Model file for the job. Use its own axes, mm. A direction names the side the tool comes from. Round coordinates to 2 decimals unless told otherwise and drop trailing zeros. Order: outer loops, then holes, each group sorted by start corner. A loop starts at its lowest first (then second) coordinate and runs counter-clockwise, first axis right, second up. Notation, with made-up numbers: (-8, 64) - (19, 64) arc R14 ccw to (19, 78) - close; hole circle Ø3 at (22, 87). An arc over 180 degrees is marked (long way). Answer as CSV lines item,"result". Start each with the question number.
1. Band-saw the part on C-C on y = -11.75. List the corners of the cut face in (x, z), then the cut area to 3 significant figures.
2. Pull direction X, two halves, no side cores. Call faces 6 (the face through (41.668, -11.944, 0.084)), 7 (the face through (-6, -4, 0)), 8 (the face through (77, -8, 0)): released by +X, released by -X, zero draft, split by the parting line, or undercut.
3. Band-saw the part on A-A on x = 85. List the corners of the cut face in (y, z).
4. Pin check, flat tips, straight feed: pin 1 Ø8 at (x, y) = (49.5, -6) entering from -Z; pin 2 Ø7.5 at (x, z) = (-2, -0.5) entering from -Y; pin 3 Ø2 at (x, z) = (60, -4) entering from +Y; pin 4 Ø12 at (x, z) = (30.5, 1) entering from +Y. Stop position of each tip, or through.
5. Band-saw the part on B-B on z = 5. List the corners of the cut face in (x, y), then the cut area to 3 significant figures.
6. Wall check: line 1 along Z through (x, y) = (85, -13.5); line 2 along Z through (x, y) = (0, -2); line 3 along Z through (x, y) = (18, -7.5). Give the ranges that are in metal, low to high. Write a range as [from, to].
7. 3-axis set-ups, long thin cutter, end or side, ignore diameter. For faces 1 (the face through (76, -16, 0)), 2 (the face through (44, -8, -6)), 3 (the face through (76.39, -12.06, 6.47)), 4 (the face through (7, -8, 0)), 5 (the face through (45, -8, 6)): which of +Z, -Z, +X, -X, +Y, -Y reach the whole face in a straight line?
8. Band-saw the part on D-D on x = 0. List the corners of the cut face in (y, z).
```python
from build123d import *

# Parameters (mm, degrees)
F0_R     = 6
F1_DEPTH = 25
F3_DEPTH = 12.5
F4_R     = 8


with BuildPart() as f1:
    # F0 (on Front) → F1 (new body)
    with BuildSketch(Plane.XZ):
        with BuildLine():
            ThreePointArc((10.965856, -6), (12.110392, -3.096514), (12.5, 0))
            ThreePointArc((12.5, 0), (12.110392, 3.096514), (10.965856, 6))
            ThreePointArc((10.965856, 6), (-12.5, 0), (10.965856, -6))
        make_face()
        Circle(F0_R, mode=Mode.SUBTRACT)
        with BuildLine():
            ThreePointArc((10.965856, 6), (12.110392, 3.096514), (12.5, 0))
            ThreePointArc((12.5, 0), (12.110392, -3.096514), (10.965856, -6))
            Line((10.965856, -6), (77, -6))
            ThreePointArc((77, -6), (75, 0), (77, 6))
            Line((77, 6), (10.965856, 6))
        make_face()
        with BuildLine():
            ThreePointArc((95, 0), (88.162278, 9.486833), (77, 6))
            ThreePointArc((77, 6), (75, 0), (77, -6))
            ThreePointArc((77, -6), (88.162278, -9.486833), (95, 0))
        make_face()
        with Locations((85, 0)):
            Circle(F0_R, mode=Mode.SUBTRACT)
    extrude(amount=F1_DEPTH)

    # F2 (on Top) → F3 (intersect, symmetric)
    with BuildSketch(Plane.XY):
        Polygon((20, 0), (-12.5, 0), (-12.5, -8), (19.300091, -8), (64.670345, -16), (95, -16), (95, -8), (65.370255, -8), align=None)
    extrude(amount=F3_DEPTH, both=True, mode=Mode.INTERSECT)

    # F4
    f4_edges = [f1.edges().sort_by_distance(p)[0] for p in [
        (10.965856, -4, -6),
        (10.965856, -4, 6),
        (77, -12, 6),
        (77, -12, -6),
    ]]
    fillet(f4_edges, radius=F4_R)


solid = f1.part
```
Reply:
1,outline,"(40.57, -6) - (73.69, -6) arc R8 cw to (78.71, -7.78) arc R10 ccw (long way) to (78.71, 7.78) arc R8 cw to (73.69, 6) - (40.57, 6) - close; hole circle Ø12 at (85, 0)"
1,area,"624 mm2"
2,face 6,"released by -X"
2,face 7,"undercut"
2,face 8,"zero draft"
3,outline,"(-16, -10) - (-8, -10) - (-8, -6) - (-16, -6) - close; (-16, 6) - (-8, 6) - (-8, 10) - (-16, 10) - close"
4,pin 1,"stops at z = -6"
4,pin 2,"passes through"
4,pin 3,"stops at y = -6.88"
4,pin 4,"stops at y = -0.79"
5,outline,"(-11.46, -8) - (-3.32, -8) - (-3.32, 0) - (-11.46, 0) - close; (3.32, -8) - (19.3, -8) - (64.67, -16) - (81.68, -16) - (81.68, -8) - (65.37, -8) - (20, 0) - (3.32, 0) - close; (88.32, -16) - (93.66, -16) - (93.66, -8) - (88.32, -8) - close"
5,area,"740 mm2"
6,line 1,"z = [-10, -6], [6, 10]"
6,line 2,"z = [-12.5, -6], [6, 12.5]"
6,line 3,"z = [-6, 6]"
7,face 1,"+Z, -Z, +X, -X, -Y"
7,face 2,"-Z, +Y, -Y"
7,face 3,"+Z, -X, +Y, -Y"
7,face 4,"+Z, -Z, -X, -Y"
7,face 5,"+Z, +Y, -Y"
8,outline,"(-8, -12.5) - (0, -12.5) - (0, -6) - (-8, -6) - close; (-8, 6) - (0, 6) - (0, 12.5) - (-8, 12.5) - close"
